Can you work these out from the drawing? Everything is in mm from the part's minimum corner. Round coordinates to 2 decimals unless told otherwise and drop trailing zeros. Loops run counter-clockwise (first coordinate to the right, second up) from the corner with the lowest first, then second, coordinate; pieces in that order, holes last. Notation, with made-up numbers: M 47,-7.5 L 73,-7.5 A13 cw 73,8.5 Z; hole C -1,14.5 d1. An arc over 180 degrees is marked long. Use a Markdown table: item, result.
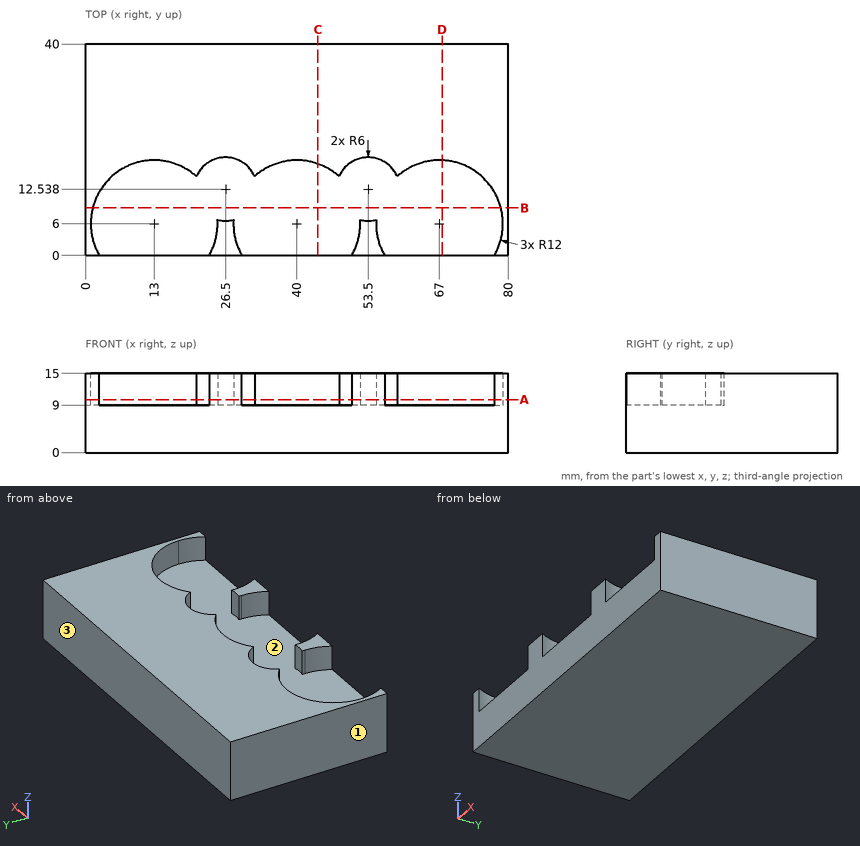
Q1. Imagine slicing it at C-C, the plane x = 44. Please give me the cut outline in (y, z), then the cut area to 3 significant figures.
Return value:
| item | result |
|---|---|
| outline | M 0,0 L 40,0 L 40,15 L 17.31,15 L 17.31,9 L 0,9 Z |
| area | 496 mm^2 |
Q2. Will this pin go through, and if not, where does the flat tip stop? P1, Ø9.5, axis at x = 38, y = 7, coming from the +Z side.
Return value:
| item | result |
|---|---|
| P1 | stops at z = 9 |
Q3. We'd pull the mould along X, two halves only. Please class the marked faces 1, 2 and 3: pulls with the +X half, pulls with the -X half, needs draft (parallel to the pull), parting line crosses it, or undercut.
Return value:
| item | result |
|---|---|
| face 1 | pulls with the -X half |
| face 2 | undercut |
| face 3 | needs draft |
Q4. Imagine slicing it at D-D, the plane x = 67.5. Please give me the cut outline in (y, z), then the cut area to 3 significant figures.
Return value:
| item | result |
|---|---|
| outline | M 0,0 L 40,0 L 40,15 L 17.99,15 L 17.99,9 L 0,9 Z |
| area | 492 mm^2 |
Q5. Imagine slicing it at A-A, the plane z = 10. Please give me the cut outline in (x, y) (1 decimal).
Return value:
| item | result |
|---|---|
| outline | M 0,0 L 2.6,0 A12 cw 21,14.9 A6 cw 32,14.9 A12 cw 48,14.9 A6 cw 59,14.9 A12 cw 77.4,0 L 80,0 L 80,40 L 0,40 Z; M 23.4,0 L 29.6,0 A12 cw 28,6.7 A6 cw 25,6.7 A12 cw Z; M 50.4,0 L 56.6,0 A12 cw 55,6.7 A6 cw 52,6.7 A12 cw Z |
Q6. I need wall thicknesses on line 1 (Z direction, x = 51, y = 4); line 2 (X direction, y = 10, z = 13.25); line 3 (Y direction, x = 50, z = 10.75). Which ranges of each line are inside material? Lowest first, please. Write a range as from..to.
Return value:
| item | result |
|---|---|
| line 1 | z = 0..9 |
| line 2 | x = 0..1.69, 78.31..80 |
| line 3 | y = 17.41..40 |
Q7. Imagine slicing it at B-B, the plane y = 9. Please give me the cut outline in (x, z).
Return value:
| item | result |
|---|---|
| outline | M 0,0 L 80,0 L 80,15 L 78.62,15 L 78.62,9 L 1.38,9 L 1.38,15 L 0,15 Z |
